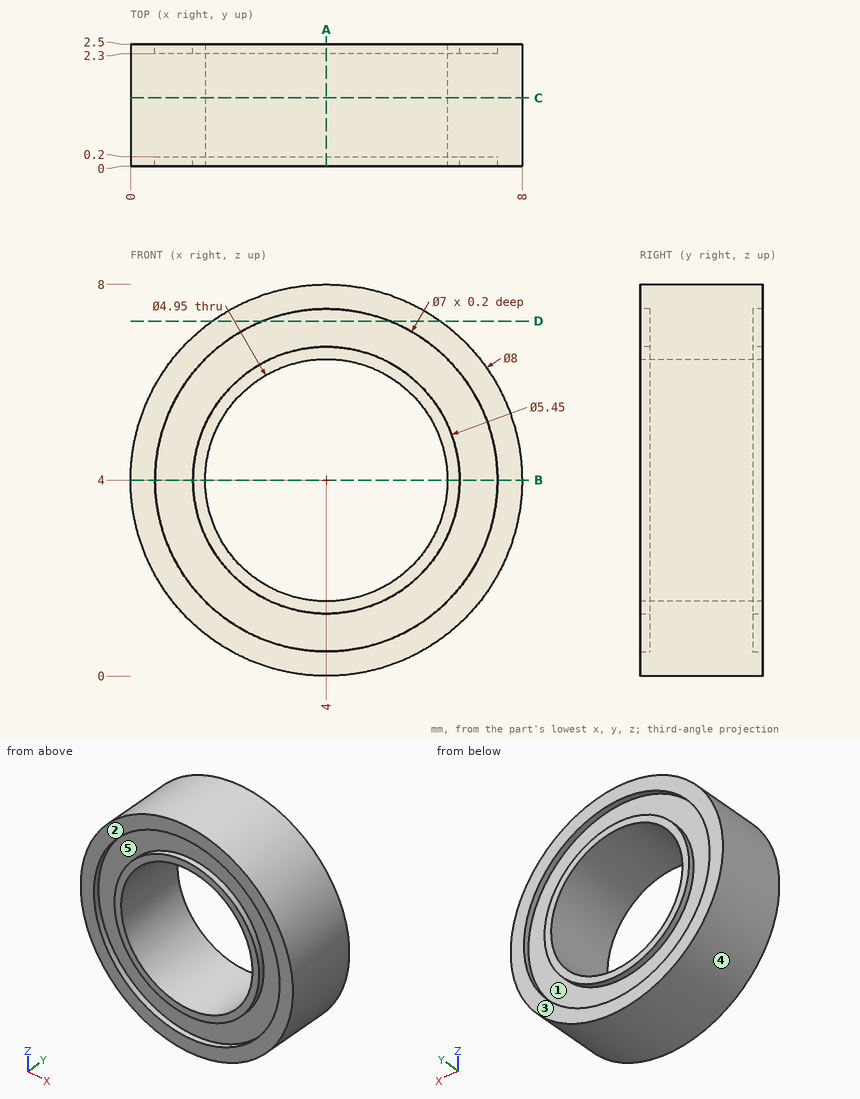
Source: three-view drawing plus pictorial views. Frame: mm from the lowest corner of the part. A direction names the side the tool comes from. Give positions to 0.01 mm unless a question says otherwise; leave off trailing zeros. Loops run counter-clockwise (first coordinate to the right, second up) from the corner with the lowest first, then second, coordinate; pieces in that order, holes last. Notation, with made-up numbers: (78.25, 66) -> (84.25, 66) arc R12 cw to (84.25, 84) -> close; hole circle Ø7 at (-24, 56). An arc over 180 degrees is marked (long way). Use a Markdown table: item, result. Add a question column.
(1) Pull-direction query (X, two-part tool) for the marked faces 3, 4 and 5; classes: +X half, -X half, draft (parallel to the pull), parting line (faces both ways), or undercut.
(2) Ray query, line 1 (X direction, y = 2.45, z = 4) (3 decimals); line 2 (X direction, y = 0.5, z = 4) (3 decimals); line 3 (Y direction, x = 5, z = 0.75). Return the intervals inside material, ascending.
(3) Section query D-D (z = 7.25). Output: boundary loops of the cut face in (x, y), then the cut area to 3 significant figures.
(4) Section query C-C (y = 1.4). Output: boundary loops of the cut face in (x, z) (3 decimals).
(5) First-contact query: pin 1 Ø1 at (x, y) = (6, 1.5) entering from -Z; pin 2 Ø1 at (x, z) = (5.5, 4) entering from +Y. Flat tips, straight axial feed; report the tip coordinate or a pass-through.
(6) Section query A-A (x = 4). Output: boundary loops of the cut face in (y, z) (3 decimals).
(7) Access query for the marked faces 1 and 2. Directions: +Z, -Z, +X, -X, +Y, -Y. A direction counts if a zero-diameter tool reaches every point of the face in a straight line with its end or side. Return the directions, or none.
(8) Section query B-B (z = 4). Output: boundary loops of the cut face in (x, y) (3 decimals).
Checked values:
| question | item | result |
|---|---|---|
| 1 | face 3 | draft |
| 1 | face 4 | parting line |
| 1 | face 5 | undercut |
| 2 | line 1 | 0 to 0.5, 1.275 to 1.525, 6.475 to 6.725, 7.5 to 8 |
| 2 | line 2 | 0 to 1.525, 6.475 to 8 |
| 2 | line 3 | 0.2 to 2.3 |
| 3 | outline | (1.67, 0) -> (2.7, 0) -> (2.7, 0.2) -> (5.3, 0.2) -> (5.3, 0) -> (6.33, 0) -> (6.33, 2.5) -> (5.3, 2.5) -> (5.3, 2.3) -> (2.7, 2.3) -> (2.7, 2.5) -> (1.67, 2.5) -> close |
| 3 | area | 10.6 mm^2 |
| 4 | outline | circle Ø8 at (4, 4); hole circle Ø4.95 at (4, 4) |
| 5 | pin 1 | z = 0.29 |
| 5 | pin 2 | through |
| 6 | outline | (0, 0) -> (2.5, 0) -> (2.5, 0.5) -> (2.3, 0.5) -> (2.3, 1.275) -> (2.5, 1.275) -> (2.5, 1.525) -> (0, 1.525) -> (0, 1.275) -> (0.2, 1.275) -> (0.2, 0.5) -> (0, 0.5) -> close; (0, 6.475) -> (2.5, 6.475) -> (2.5, 6.725) -> (2.3, 6.725) -> (2.3, 7.5) -> (2.5, 7.5) -> (2.5, 8) -> (0, 8) -> (0, 7.5) -> (0.2, 7.5) -> (0.2, 6.725) -> (0, 6.725) -> close |
| 7 | face 1 | +Y |
| 7 | face 2 | +Z, -Z, +X, -X, -Y |
| 8 | outline | (0, 0) -> (0.5, 0) -> (0.5, 0.2) -> (1.275, 0.2) -> (1.275, 0) -> (1.525, 0) -> (1.525, 2.5) -> (1.275, 2.5) -> (1.275, 2.3) -> (0.5, 2.3) -> (0.5, 2.5) -> (0, 2.5) -> close; (6.475, 0) -> (6.725, 0) -> (6.725, 0.2) -> (7.5, 0.2) -> (7.5, 0) -> (8, 0) -> (8, 2.5) -> (7.5, 2.5) -> (7.5, 2.3) -> (6.725, 2.3) -> (6.725, 2.5) -> (6.475, 2.5) -> close |
